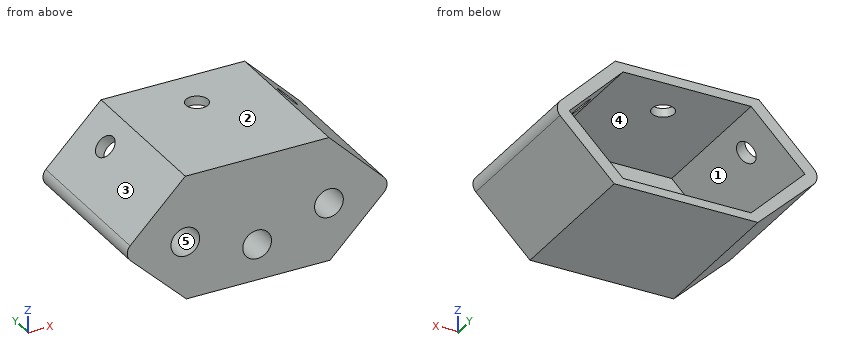
```python
from build123d import *

# Parameters (mm, degrees)
RESSALTO_EXTRUS_O3_DEPTH  = 25
ESBO_O4_W                 = 17.1
ESBO_O4_H                 = 14.6
CORTE_EXTRUS_O1_DEPTH     = 23.8
ESBO_O5_R                 = 1.95
CORTE_EXTRUS_O2_DEPTH     = 23.8
CORTE_EXTRUS_O3_DEPTH     = 23.8
RESSALTO_EXTRUS_O11_START = 4
ESBO_O9_R                 = 2.35
ESBO_O9_R_2               = 1.95
ESBO_O9_R_3               = 2.468896698
RESSALTO_EXTRUS_O11_DEPTH = 4
ESBO_O11_W                = 83.094173182
ESBO_O11_H                = 8
CORTE_EXTRUS_O10_DEPTH    = 30
ESBO_O19_R                = 1.5
CORTE_EXTRUS_O12_DEPTH    = 30
ESBO_O22_R                = 1.5
CORTE_EXTRUS_O13_DEPTH    = 30
ESBO_O23_R                = 1.5
CORTE_EXTRUS_O14_DEPTH    = 30


with BuildPart() as part:
    # Esbo_o1 → Ressalto-extrus_o3 (new body)
    with BuildSketch(Plane(origin=(0, 0, 0), x_dir=(1, 0, 0), z_dir=(0, 1, 0))):
        with BuildLine():
            Line((9.888111981, 8.359296796), (-9.611888019, 8.359296796))
            Line((-9.611888019, 8.359296796), (-17.250307666, 0.999703565))
            ThreePointArc((-17.250307666, 0.999703565), (-17.631966883, 0.000271602), (-17.250692692, -0.999307308))
            Line((-17.250692692, -0.999307308), (-9.75, -8.5))
            Line((-9.75, -8.5), (9.75, -8.5))
            Line((9.75, -8.5), (17.25, -1))
            ThreePointArc((17.25, -1), (17.631966011, 0), (17.25, 1))
            Line((17.25, 1), (9.888111981, 8.359296796))
        make_face()
    extrude(amount=RESSALTO_EXTRUS_O3_DEPTH)

    # Esbo_o4 → Corte-extrus_o1 (cut)
    with BuildSketch(Plane(origin=(0, 25, 0), x_dir=(1, 0, 0), z_dir=(0, 1, 0))):
        Polygon((-15.85, 0), (-8.55, 7.3), (-8.55, -7.3), align=None)
        Rectangle(ESBO_O4_W, ESBO_O4_H)
        Polygon((8.55, 7.3), (15.85, 0), (8.55, -7.3), align=None)
    extrude(amount=-CORTE_EXTRUS_O1_DEPTH, mode=Mode.SUBTRACT)

    # Esbo_o5 → Corte-extrus_o2 (cut)
    with BuildSketch(Plane(origin=(0, 1.2, 0), x_dir=(1, 0, 0), z_dir=(0, 1, 0))):
        with Locations(Location((0, 3.5, 0), (0, 0, 270))):
            Circle(ESBO_O5_R)
        with Locations(Location((-9.75, 0.5, 0), (0, 0, 270))):
            Circle(ESBO_O5_R)
        with Locations(Location((9.75, 0.5, 0), (0, 0, 270))):
            Circle(ESBO_O5_R)
    extrude(amount=-CORTE_EXTRUS_O2_DEPTH, mode=Mode.SUBTRACT)

    # Esbo_o7 → Corte-extrus_o3 (cut)
    with BuildSketch(Plane(origin=(0, 25, 0), x_dir=(1, 0, 0), z_dir=(0, 1, 0))):
        Polygon((-15.85, 0), (-8.55, 7.3), (-8.691421356, 7.3), (-15.920710678, 0.070710678), align=None)
        Polygon((-8.55, -7.3), (-15.85, 0), (-15.920710678, 0.070710678), (-15.991421356, 0), (-8.691421356, -7.3), align=None)
        Polygon((8.691421356, -7.3), (8.55, -7.3), (15.85, 0), (8.55, 7.3), (8.691421356, 7.3), (15.991421356, 0), align=None)
    extrude(amount=-CORTE_EXTRUS_O3_DEPTH, mode=Mode.SUBTRACT)

    # Esbo_o9 → Ressalto-extrus_o11 (add)
    # profile 1 of 3: a face of its own
    with BuildSketch(Plane(origin=(0, 1.2, 0), x_dir=(1, 0, 0), z_dir=(0, 1, 0)).offset(RESSALTO_EXTRUS_O11_START)):
        with Locations(Location((-9.75, 0.5, 0), (0, 0, 270))):
            Circle(ESBO_O9_R)
        with Locations(Location((-9.75, 0.5, 0), (0, 0, 270))):
            Circle(ESBO_O9_R_2, mode=Mode.SUBTRACT)
    # profile 2 of 3: a face of its own
    with BuildSketch(Plane(origin=(0, 1.2, 0), x_dir=(1, 0, 0), z_dir=(0, 1, 0)).offset(RESSALTO_EXTRUS_O11_START)):
        with Locations(Location((0, 3.5, 0), (0, 0, 270))):
            Circle(ESBO_O9_R_3)
        with Locations(Location((0, 3.5, 0), (0, 0, 270))):
            Circle(ESBO_O9_R_2, mode=Mode.SUBTRACT)
    # profile 3 of 3: a face of its own
    with BuildSketch(Plane(origin=(0, 1.2, 0), x_dir=(1, 0, 0), z_dir=(0, 1, 0)).offset(RESSALTO_EXTRUS_O11_START)):
        with Locations(Location((9.75, 0.5, 0), (0, 0, 270))):
            Circle(ESBO_O9_R)
        with Locations(Location((9.75, 0.5, 0), (0, 0, 270))):
            Circle(ESBO_O9_R_2, mode=Mode.SUBTRACT)
    extrude(amount=-RESSALTO_EXTRUS_O11_DEPTH)

    # Esbo_o11 → Corte-extrus_o10 (cut)
    with BuildSketch(Plane.XY.offset(8.5)):
        with Locations((0, 25)):
            Rectangle(ESBO_O11_W, ESBO_O11_H)
    extrude(amount=-CORTE_EXTRUS_O10_DEPTH, mode=Mode.SUBTRACT)

    # Esbo_o19 → Corte-extrus_o12 (cut)
    with BuildSketch(Plane(origin=(7.995710678, 0, 7.995710678), x_dir=(-0.7071067811865476, 0, 0.7071067811865476), z_dir=(-0.7071067811865476, 0, -0.7071067811865476))):
        with Locations((-4.483883476, 15)):
            Circle(ESBO_O19_R)
    extrude(amount=-CORTE_EXTRUS_O12_DEPTH, mode=Mode.SUBTRACT)

    # Esbo_o22 → Corte-extrus_o13 (cut)
    with BuildSketch(Plane(origin=(0, 0, 7.3), x_dir=(-1, 0, 0), z_dir=(0, 0, -1))):
        with Locations((0, 15)):
            Circle(ESBO_O22_R)
    extrude(amount=-CORTE_EXTRUS_O13_DEPTH, mode=Mode.SUBTRACT)

    # Esbo_o23 → Corte-extrus_o14 (cut)
    with BuildSketch(Plane(origin=(-7.995710678, 0, 7.995710678), x_dir=(-0.7071067811865476, 0, -0.7071067811865475), z_dir=(0.7071067811865475, 0, -0.7071067811865476))):
        with Locations((4.683883476, 15)):
            Circle(ESBO_O23_R)
    extrude(amount=-CORTE_EXTRUS_O14_DEPTH, mode=Mode.SUBTRACT)


solid = part.part
```
Model file for the job. Use its own axes, mm. Face numbers are marked on the shaded views. A direction names the side the tool comes from. Round coordinates to 2 decimals unless told otherwise and drop trailing zeros. Write each loop counter-clockwise with the first axis right and the second up, starting at its lowest first coordinate (ties: lowest second). Pieces come first, ordered by that corner, then holes. Notation, with made-up numbers: (14.25, 11.25) - (25.25, 11.25) arc R24 cw to (25.25, 36.25) - close; hole circle Ø3 at (71.25, 6.25). An arc over 180 degrees is marked (long way). One line per item, written item: value.
(1) Drop flat-ended pins along their axis: P1, Ø3, axis at x = -9.75, z = -0.5, coming from the -Y side; P2, Ø3, axis at x = -12, z = -1, coming from the +Y side; P3, Ø1, axis at y = 16, z = -2, coming from the -X side. Give the stop position or say it passes through.
Values follow:
P1: passes through
P2: stops at y = 5.2
P3: stops at x = -16.73
(2) Cut at B-B, the plane z = -3.5. Give the cut face in (x, y), plus the area to 3 significant figures.
Values follow:
outline: (-14.66, 0) - (-1.95, 0) - (-1.95, 5.2) - (-2.47, 5.2) - (-2.47, 1.2) - (-12.49, 1.2) - (-12.49, 21) - (-14.66, 21) - close; (1.95, 0) - (14.75, 0) - (14.75, 21) - (12.49, 21) - (12.49, 1.2) - (2.47, 1.2) - (2.47, 5.2) - (1.95, 5.2) - close
area: 122 mm²
(3) Two-plate mould, pull along X, no slides. Class the marked faces 1, 2 and 3: pulls with the +X half, pulls with the -X half, needs draft (parallel to the pull), parting line crosses it, or undercut.
Values follow:
face 1: undercut
face 2: needs draft
face 3: pulls with the -X half
(4) 3-axis set-ups, long thin cutter, end or side, ignore diameter. For the marked faces 4 and 5: which of +Z, -Z, +X, -X, +Y, -Y reach the whole face in a straight line?
Values follow:
face 4: +Y
face 5: +Y, -Y
(5) Wall check: probe 1 along Z at (x, y) = (-1.5, 17.25); probe 2 along X at (y, z) = (2.1, -0.5); probe 3 along Y at (x, z) = (-2, 7.25). Give the ranges that are in metal, low to high.
Values follow:
probe 1: z = -8.36 to -7.3, 7.3 to 8.5
probe 2: x = -17.55 to -15.49, -12.1 to -11.7, -7.8 to -7.4, 7.4 to 7.8, 11.7 to 12.1, 15.49 to 17.55
probe 3: y = 0 to 1.2
(6) Cut at C-C, the plane y = 7.5. Give the cut face in (x, z).
Values follow:
outline: (-17.25, -1) - (-9.61, -8.36) - (9.89, -8.36) - (17.25, -1) arc R1.5 ccw to (17.25, 1) - (9.75, 8.5) - (-9.75, 8.5) - (-17.25, 1) arc R1.5 ccw to start; hole (-15.99, 0) - (-8.69, -7.3) - (8.69, -7.3) - (15.99, 0) - (8.69, 7.3) - (-8.69, 7.3) - close
(7) Cut at A-A, the plane x = 0. Give the cut face in (y, z), plus the area to 3 significant figures.
Values follow:
outline: (0, -8.36) - (21, -8.36) - (21, -7.3) - (1.2, -7.3) - (1.2, -5.97) - (5.2, -5.97) - (5.2, -5.45) - (0, -5.45) - close; (0, -1.55) - (5.2, -1.55) - (5.2, -1.03) - (1.2, -1.03) - (1.2, 7.3) - (13.5, 7.3) - (13.5, 8.5) - (0, 8.5) - close; (16.5, 7.3) - (21, 7.3) - (21, 8.5) - (16.5, 8.5) - close
area: 60.8 mm²
(8) Cut at D-D, the plane y = 15. Give the cut face in (x, z).
Values follow:
outline: (-17.25, -1) - (-9.61, -8.36) - (9.89, -8.36) - (17.25, -1) arc R1.5 ccw to (17.25, 1) - (13.36, 4.89) - (12.23, 3.76) - (15.99, 0) - (8.69, -7.3) - (-8.69, -7.3) - (-15.99, 0) - (-12.37, 3.62) - (-13.5, 4.75) - (-17.25, 1) arc R1.5 ccw to start; (-11.38, 6.87) - (-10.25, 5.74) - (-8.69, 7.3) - (-1.5, 7.3) - (-1.5, 8.5) - (-9.75, 8.5) - close; (1.5, 7.3) - (8.69, 7.3) - (10.11, 5.89) - (11.23, 7.02) - (9.75, 8.5) - (1.5, 8.5) - close
